from build123d import *

# Parameters (mm, degrees)
F1_DEPTH = 25.4
F2_DEPTH = 50.8
F3_R     = 10.0458196752
F4_DEPTH = 203.2


# Not quite as in the source:
# - the program builds the solid bodies; features that only make, move or delete a surface that nothing else refers to are left out


with BuildPart() as f1:
    # F0 (on Top) → F1 (new body)
    with BuildSketch(Plane.XY):
        Polygon((28.6761522293, 32.8064598143), (-34.5765948296, 32.8064598143), (-55.3461499512, -32.0984050632), (52.9859773815, -32.0984050632), align=None)
    extrude(amount=F1_DEPTH)

    # F2 (add): a face of the model
    f2_faces = [f1.faces().sort_by_distance(p)[0] for p in [
        (-1.9876444454, -2.4879782653, 0),
    ]]
    extrude(f2_faces, amount=F2_DEPTH)

    # F3 (on Front) → F4 (join)
    with BuildSketch(Plane.XZ):
        with Locations((0, -11.2053733319)):
            Circle(F3_R)
    extrude(amount=-F4_DEPTH)


solid = f1.part
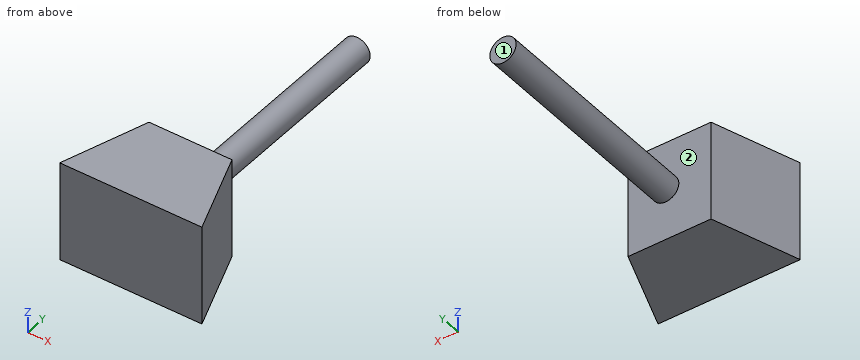
CAD build for the part. Positions are in the model's coordinates, mm. Face numbers are marked on the shaded views. A direction names the side the tool comes from. Give positions to 0.01 mm unless a question says otherwise; leave off trailing zeros. Order: outer loops, then holes, each group sorted by start corner. A loop starts at its lowest first (then second) coordinate and runs counter-clockwise, first axis right, second up. Notation, with made-up numbers: (65, 41) - (115, 41) arc R8 ccw to (115, 54) - close; hole circle Ø5 at (-15, 10.25). An arc over 180 degrees is marked (long way). Answer in a Markdown table with one row per item.
1. Saw through at D-D, the plane y = 111.5. Give the cut face in (x, z).
Data:
| item | result |
|---|---|
| outline | circle Ø20.09 at (0, -11.21) |
2. Saw through at C-C, the plane x = 14. Give the cut face in (y, z), plus the area to 3 significant figures.
Data:
| item | result |
|---|---|
| outline | (-32.1, -50.8) - (32.81, -50.8) - (32.81, 25.4) - (-32.1, 25.4) - close |
| area | 4,950 mm² |
3. Flat gauge pins, fed straight in: pin 1 (5 mm diameter, centred on y = 133.5, z = -25.5, fed in from -X); pin 2 (6 mm diameter, centred on x = -34, z = 9.5, fed in from +Y). Where does each tip first touch, or does it go through?
Data:
| item | result |
|---|---|
| pin 1 | passes through |
| pin 2 | stops at y = 32.81 |
4. Tool access for the marked faces 1 and 2: list every direction of +Z, -Z, +X, -X, +Y, -Y with a clear straight run to the whole face (end or side of a thin tool).
Data:
| item | result |
|---|---|
| face 1 | +Z, -Z, +X, -X, +Y |
| face 2 | +Y |
5. Saw through at B-B, the plane z = -39. Give the cut face in (x, y), plus the area to 3 significant figures.
Data:
| item | result |
|---|---|
| outline | (-55.35, -32.1) - (52.99, -32.1) - (28.68, 32.81) - (-34.58, 32.81) - close |
| area | 5,570 mm² |
6. Saw through at A-A, the plane x = 0. Give the cut face in (y, z), plus the area to 3 significant figures.
Data:
| item | result |
|---|---|
| outline | (-32.1, -50.8) - (32.81, -50.8) - (32.81, -21.25) - (203.2, -21.25) - (203.2, -1.16) - (32.81, -1.16) - (32.81, 25.4) - (-32.1, 25.4) - close |
| area | 8,370 mm² |
7. Probe probe 1 along Y at (x, z) = (-33.5, 9.5); probe 2 along X at (y, z) = (170, -19); probe 3 along X at (y, z) = (-1.5, -30.5). List the from-to ranges inside material, lowest first. Write a range as [from, to].
Data:
| item | result |
|---|---|
| probe 1 | y = [-32.1, 32.81] |
| probe 2 | x = [-6.34, 6.34] |
| probe 3 | x = [-45.55, 41.53] |
